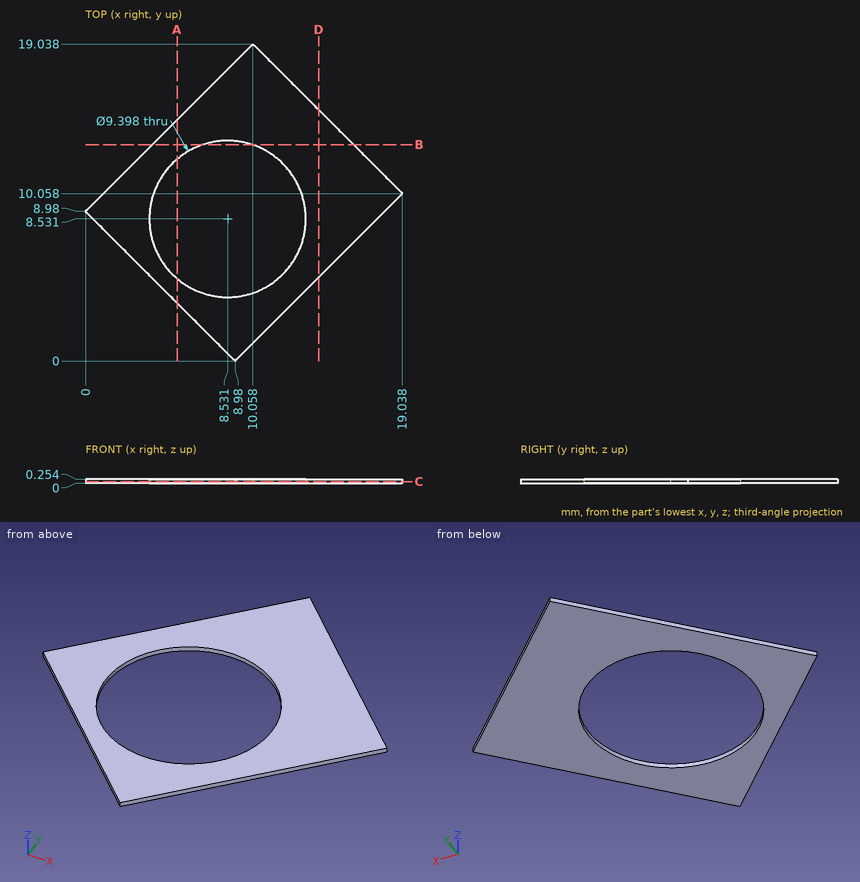
Verification items for this drawing (mm, ordinates from the low corner). Round coordinates to 2 decimals unless told otherwise and drop trailing zeros. Loops run counter-clockwise (first coordinate to the right, second up) from the corner with the lowest first, then second, coordinate; pieces in that order, holes last. Notation, with made-up numbers: (56.25, -5) -> (66.25, -5) arc R18 ccw to (66.25, 8) -> close; hole circle Ø10 at (-1, 14). An arc over 180 degrees is marked (long way). Answer in a Markdown table with one row per item.
Q1. Sectioned sample at C-C on z = 0.1. Enter the section's corners in (x, y).
Data:
| item | result |
|---|---|
| outline | (0, 8.98) -> (8.98, 0) -> (19.04, 10.06) -> (10.06, 19.04) -> close; hole circle Ø9.4 at (8.53, 8.53) |
Q2. Sectioned sample at A-A on x = 5.5. Enter the section's corners in (y, z).
Data:
| item | result |
|---|---|
| outline | (3.48, 0) -> (4.94, 0) -> (4.94, 0.25) -> (3.48, 0.25) -> close; (12.12, 0) -> (14.48, 0) -> (14.48, 0.25) -> (12.12, 0.25) -> close |
Q3. Sectioned sample at D-D on x = 14. Enter the section's corners in (y, z).
Data:
| item | result |
|---|---|
| outline | (5.02, 0) -> (15.1, 0) -> (15.1, 0.25) -> (5.02, 0.25) -> close |
Q4. Thickness scan on L1, parallel to Y at x = 4.25, z = 0.15 (1 decimal); L2, parallel to X at y = 9, z = 0.2 (1 decimal); L3, parallel to Y at x = 5.75, z = 0.2 (1 decimal). Record the ranges inside material, lowest first.
Data:
| item | result |
|---|---|
| L1 | y = 4.7 to 6.6, 10.5 to 13.2 |
| L2 | x = 0 to 3.9, 13.2 to 18 |
| L3 | y = 3.2 to 4.7, 12.3 to 14.7 |
Q5. Sectioned sample at B-B on y = 13. Enter the section's corners in (x, z).
Data:
| item | result |
|---|---|
| outline | (4.02, 0) -> (7.08, 0) -> (7.08, 0.25) -> (4.02, 0.25) -> close; (9.98, 0) -> (16.1, 0) -> (16.1, 0.25) -> (9.98, 0.25) -> close |
